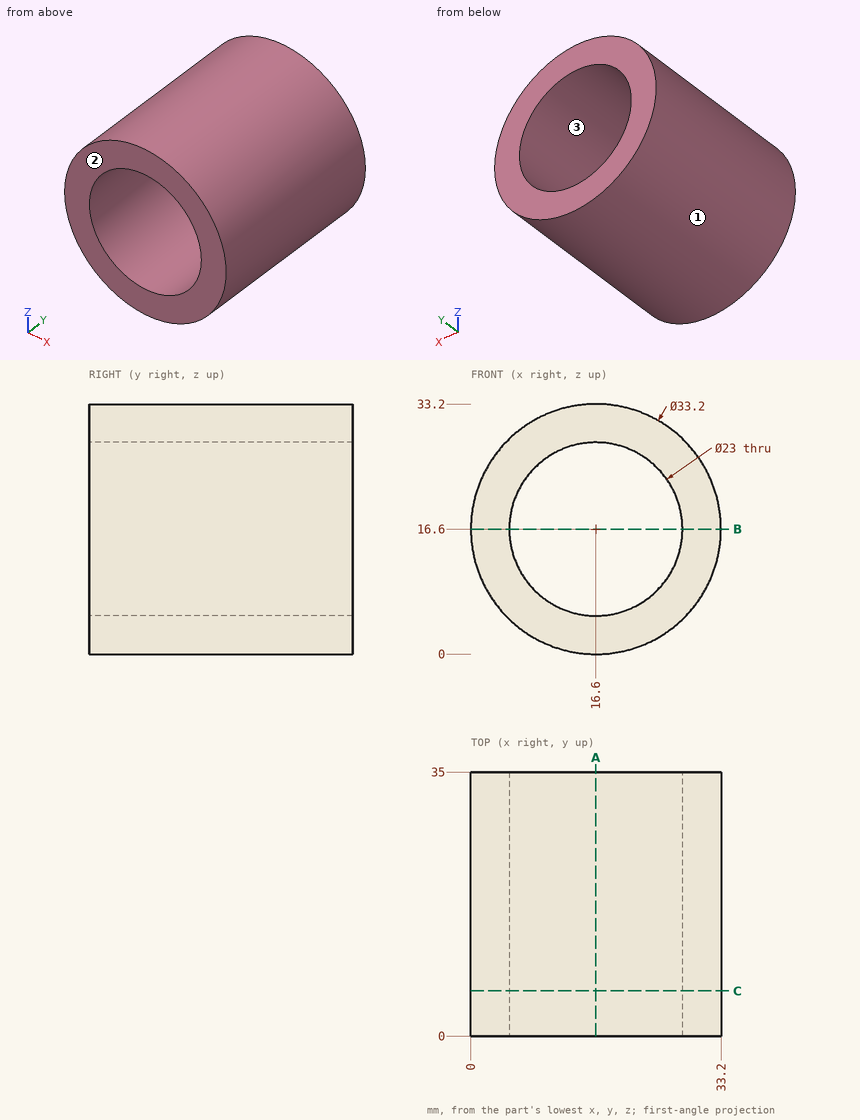
Could you check a few things on this drawing? It's one solid part, dimensions in mm from its lowest x, y, z. Give positions to 0.01 mm unless a question says otherwise; leave off trailing zeros. Write each loop counter-clockwise with the first axis right and the second up, starting at its lowest first coordinate (ties: lowest second). Pieces come first, ordered by that corner, then holes. Notation, with made-up numbers: (48, 2) -> (59, 2) arc R12 cw to (59, 17) -> close; hole circle Ø1 at (-12.75, 60.5). An arc over 180 degrees is marked (long way). Answer as a JSON object with one key per item and string values.
Q1. Suppose I cut it at A-A on x = 16.6. Write out the boundary of the cut face in (y, z), then the cut area to 3 significant figures.
Taken from the geometry:
{"outline": "(0, 0) -> (35, 0) -> (35, 5.1) -> (0, 5.1) -> close; (0, 28.1) -> (35, 28.1) -> (35, 33.2) -> (0, 33.2) -> close", "area": "357 mm²"}
Q2. Please list where these lines run through material, in increasing order: L1, parallel to Z at x = 16.6, y = 9; L2, parallel to Z at x = 22, y = 22.5; L3, parallel to X at y = 7.5, z = 24.
Taken from the geometry:
{"L1": "z = 0 to 5.1, 28.1 to 33.2", "L2": "z = 0.9 to 6.45, 26.75 to 32.3", "L3": "x = 1.74 to 7.8, 25.4 to 31.46"}
Q3. Suppose I cut it at B-B on z = 16.6. Write out the boundary of the cut face in (x, y).
Taken from the geometry:
{"outline": "(0, 0) -> (5.1, 0) -> (5.1, 35) -> (0, 35) -> close; (28.1, 0) -> (33.2, 0) -> (33.2, 35) -> (28.1, 35) -> close"}
Q4. We'd pull the mould along X, two halves only. Please class the marked faces 1, 2 and 3: released by +X, released by -X, zero draft, split by the parting line, or undercut.
Taken from the geometry:
{"face 1": "split by the parting line", "face 2": "zero draft", "face 3": "undercut"}
Q5. Suppose I cut it at C-C on y = 6. Write out the boundary of the cut face in (x, z), then the cut area to 3 significant figures.
Taken from the geometry:
{"outline": "circle Ø33.2 at (16.6, 16.6); hole circle Ø23 at (16.6, 16.6)", "area": "450 mm²"}
Q6. Will these pins go through, and if not, where does the flat tip stop? pin 1 Ø6 at (x, z) = (25.5, 4) entering from -Y; pin 2 Ø5 at (y, z) = (3.5, 24) entering from +X; pin 3 Ø2 at (x, y) = (14.5, 20) entering from +Z; pin 4 Ø1.5 at (y, z) = (27.5, 21.5) entering from +X.
Taken from the geometry:
{"pin 1": "stops at y = 0", "pin 2": "stops at x = 32.46", "pin 3": "stops at z = 33.16", "pin 4": "stops at x = 32.67"}
